Could you check a few things on this drawing? It's one solid part, dimensions in mm from its lowest x, y, z. A direction names the side the tool comes from. Give positions to 0.01 mm unless a question says otherwise; leave off trailing zeros. Write each loop counter-clockwise with the first axis right and the second up, starting at its lowest first coordinate (ties: lowest second). Pieces come first, ordered by that corner, then holes. Notation, with made-up numbers: M -25.75,80.5 L 28.25,80.5 A21 cw 28.25,91.5 Z; hole C 15.5,13.5 d1. An arc over 180 degrees is marked long. Write each question's results on one line, items separated by ' | '. Start each with the question number.
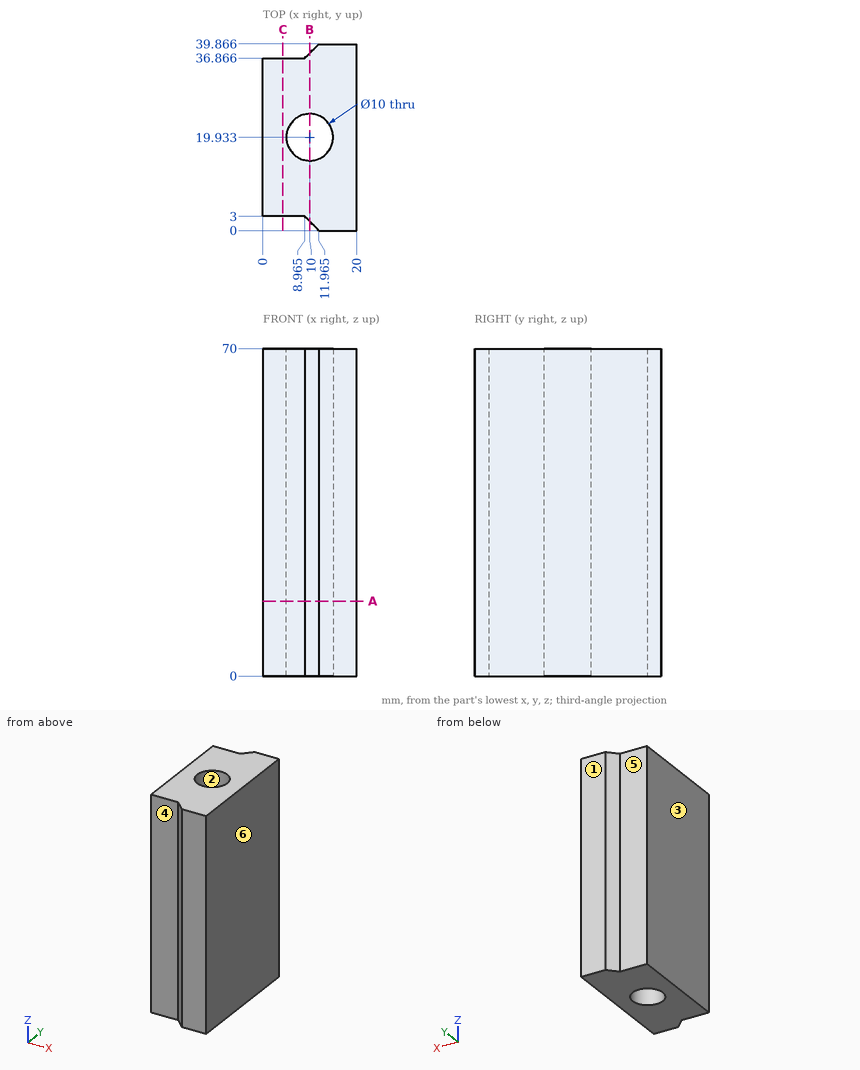
Q1. Please list where these lines run through material, in increasing order: line 1 (X direction, y = 20, z = 6); line 2 (X direction, y = 17.5, z = 35); line 3 (Y direction, x = 13, z = 44.5) (1 decimal). Write a range as [from, to].
Q2. If we section it at A-A (z = 16): Please give me the cut outline in (x, y) (1 decimal), plus the area to 3 significant figures.
Q3. If we section it at C-C (x = 4.25): Please give me the cut outline in (y, z).
Q4. For the marked faces 4, 5 and 6, which set-ups out of +Z, -Z, +X, -X, +Y, -Y let a thin tool reach every point of the face, with its end or its side?
Q5. If we section it at B-B (x = 10): Please give me the cut outline in (y, z) (1 decimal), plus the area to 3 significant figures.
Q6. I'm going to push flat-ended pins straight in: P1, Ø1.5, axis at x = 4.5, z = 12, coming from the +Y side; P2, Ø4.5, axis at x = 3, z = 33, coming from the -Y side. Where does each tip first touch, or does it pass through?
Q7. If we mould it in two halves opening along X, with no side actions, what happens to the marked faces 1, 2 and 3? For each: pulls with the +X half, pulls with the -X half, needs draft (parallel to the pull), parting line crosses it, or undercut.
Determined:
1) line 1: x = [0, 5], [15, 20] | line 2: x = [0, 5.63], [14.37, 20] | line 3: y = [0, 15.9], [23.9, 39.9]
2) outline: M 0,3 L 9,3 L 12,0 L 20,0 L 20,39.9 L 12,39.9 L 9,36.9 L 0,36.9 Z; hole C 10,19.9 d10 | area: 656 mm²
3) outline: M 3,0 L 36.87,0 L 36.87,70 L 3,70 Z
4) face 4: +Z, -Z, -X, -Y | face 5: +Z, -Z, -X, +Y | face 6: +Z, -Z, +X, +Y, -Y
5) outline: M 2,0 L 14.9,0 L 14.9,70 L 2,70 Z; M 24.9,0 L 37.9,0 L 37.9,70 L 24.9,70 Z | area: 1,820 mm²
6) P1: stops at y = 36.87 | P2: stops at y = 3
7) face 1: needs draft | face 2: undercut | face 3: pulls with the -X half
